Here's how the part is built. I have some questions about the finished solid (model axes, mm). A direction names the side the tool comes from. Give positions to 0.01 mm unless a question says otherwise; leave off trailing zeros. Order: outer loops, then holes, each group sorted by start corner. A loop starts at its lowest first (then second) coordinate and runs counter-clockwise, first axis right, second up.
from build123d import *

# Parameters (mm, degrees)
F0_W         = 40.64
F0_H         = 5.08
F1_DEPTH     = 6.35
F3_DEPTH     = 7.62
F4_R         = 1.26999
F5_T1_DEPTH  = 6.35
F5_T3_DEPTH  = 85.09
F5_T5_DEPTH  = 72.39
F5_T8_ANGLE  = 90
F5_T10_ANGLE = 90
F5_T12_ANGLE = 90
F5_T14_ANGLE = 90
F6_R         = 5.07999
F7_R         = 2.54


# Not quite as in the source:
# - a fillet or chamfer that OpenCascade refuses, or shapes differently, is made with other operations: its cross-section is extruded or revolved along the edge and cut away or added
# - a fillet or chamfer is up to 0.001 mm smaller than in the source, because OpenCascade refuses the exact size


with BuildPart() as f1:
    # F0 (on Front) → F1 (new body)
    with BuildSketch(Plane.XZ):
        with BuildLine():
            ThreePointArc((-31.75, 19.05), (-45.2203841816, 13.4703841816), (-50.8, 0))
            Line((-50.8, 0), (-50.8, -6.35))
            ThreePointArc((-50.8, -6.35), (-48.9401280605, -10.8401280605), (-44.45, -12.7))
            Line((-44.45, -12.7), (27.94, -12.7))
            Line((27.94, -12.7), (27.94, 19.05))
            Line((27.94, 19.05), (20.32, 19.05))
            Line((20.32, 19.05), (-31.75, 19.05))
        make_face()
        Rectangle(F0_W, F0_H, mode=Mode.SUBTRACT)
    extrude(amount=F1_DEPTH)

    # F2 (on face) → F3 (join)
    with BuildSketch(Plane.YZ.offset(27.94)):
        Polygon((-4.445, -5.715), (-3.175, -5.715), (-1.905, -5.715), (-1.905, 12.065), (-4.445, 12.065), align=None)
    extrude(amount=F3_DEPTH)

    # F4 (radius 1.27 in the source; OpenCascade refuses exactly that, so slightly less here)
    f4_edges = [f1.edges().sort_by_distance(p)[0] for p in [
        (35.56, -4.445, 3.175),
        (35.56, -3.175, 12.065),
        (35.56, -1.905, 3.175),
        (35.56, -3.175, -5.715),
    ]]
    fillet(f4_edges, radius=F4_R)

    # F5: fillet of radius 5.08 on 2 edges, made by hand

    # F5_s2 → F5_t1 (cut)
    with BuildSketch(Plane.XY.offset(-6.35)):
        with BuildLine():
            ThreePointArc((-45.72, 0), (-49.3121024484, -1.4878975516), (-50.8, -5.08))
            Line((-50.8, -5.08), (-50.8, 0))
            Line((-50.8, 0), (-45.72, 0))
        make_face()
        with BuildLine():
            ThreePointArc((-45.72, -6.35), (-49.3121024484, -4.8621024484), (-50.8, -1.27))
            Line((-50.8, -1.27), (-50.8, -6.35))
            Line((-50.8, -6.35), (-45.72, -6.35))
        make_face()
    extrude(amount=F5_T1_DEPTH, mode=Mode.SUBTRACT)

    # F5_s4 → F5_t3 (cut)
    with BuildSketch(Plane.YZ.offset(-44.45)):
        with BuildLine():
            ThreePointArc((-5.08, -12.7), (-1.4878975516, -11.2121024484), (0, -7.62))
            Line((0, -7.62), (0, -12.7))
            Line((0, -12.7), (-5.08, -12.7))
        make_face()
        with BuildLine():
            ThreePointArc((-1.27, -12.7), (-4.8621024484, -11.2121024484), (-6.35, -7.62))
            Line((-6.35, -7.62), (-6.35, -12.7))
            Line((-6.35, -12.7), (-1.27, -12.7))
        make_face()
    extrude(amount=F5_T3_DEPTH, mode=Mode.SUBTRACT)

    # F5_s6 → F5_t5 (cut)
    with BuildSketch(Plane.YZ.offset(-31.75)):
        with BuildLine():
            ThreePointArc((0, 13.97), (-1.4878975516, 17.5621024484), (-5.08, 19.05))
            Line((-5.08, 19.05), (0, 19.05))
            Line((0, 19.05), (0, 13.97))
        make_face()
        with BuildLine():
            ThreePointArc((-6.35, 13.97), (-4.8621024484, 17.5621024484), (-1.27, 19.05))
            Line((-1.27, 19.05), (-6.35, 19.05))
            Line((-6.35, 19.05), (-6.35, 13.97))
        make_face()
    extrude(amount=F5_T5_DEPTH, mode=Mode.SUBTRACT)

    # F5_s7 → F5_t8 (revolve, cut)
    with BuildSketch(Plane.XY.offset(-6.35)):
        with BuildLine():
            ThreePointArc((-45.72, -6.35), (-49.3121024484, -4.8621024484), (-50.8, -1.27))
            Line((-50.8, -1.27), (-50.8, -6.35))
            Line((-50.8, -6.35), (-45.72, -6.35))
        make_face()
    revolve(axis=Axis((-44.45, -6.35, -6.35), (0, -1, 0)), revolution_arc=F5_T8_ANGLE, mode=Mode.SUBTRACT)

    # F5_s9 → F5_t10 (revolve, cut)
    with BuildSketch(Plane.YZ.offset(-31.75)):
        with BuildLine():
            ThreePointArc((0, 13.97), (-1.4878975516, 17.5621024484), (-5.08, 19.05))
            Line((-5.08, 19.05), (0, 19.05))
            Line((0, 19.05), (0, 13.97))
        make_face()
    revolve(axis=Axis((-31.75, 0, 0), (0, -1, 0)), revolution_arc=F5_T10_ANGLE, mode=Mode.SUBTRACT)

    # F5_s11 → F5_t12 (revolve, cut)
    with BuildSketch(Plane.XY.offset(-6.35)):
        with BuildLine():
            ThreePointArc((-45.72, 0), (-49.3121024484, -1.4878975516), (-50.8, -5.08))
            Line((-50.8, -5.08), (-50.8, 0))
            Line((-50.8, 0), (-45.72, 0))
        make_face()
    revolve(axis=Axis((-44.45, 0, -6.35), (0, -1, 0)), revolution_arc=F5_T12_ANGLE, mode=Mode.SUBTRACT)

    # F5_s13 → F5_t14 (revolve, cut)
    with BuildSketch(Plane.YZ.offset(-31.75)):
        with BuildLine():
            ThreePointArc((-6.35, 13.97), (-4.8621024484, 17.5621024484), (-1.27, 19.05))
            Line((-1.27, 19.05), (-6.35, 19.05))
            Line((-6.35, 19.05), (-6.35, 13.97))
        make_face()
    revolve(axis=Axis((-31.75, -6.35, 0), (0, -1, 0)), revolution_arc=F5_T14_ANGLE, mode=Mode.SUBTRACT)

    # F6 (radius 5.08 in the source; OpenCascade refuses exactly that, so slightly less here)
    f6_edges = [f1.edges().sort_by_distance(p)[0] for p in [
        (20.32, -3.175, -2.54),
    ]]
    fillet(f6_edges, radius=F6_R)

    # F7
    f7_edges = [f1.edges().sort_by_distance(p)[0] for p in [
        (-20.32, -3.175, -2.54),
    ]]
    fillet(f7_edges, radius=F7_R)


solid = f1.part
Q1. I need wall thicknesses on L1, parallel to X at y = -3.25, z = -1; L2, parallel to Z at x = 31, y = -2 (3 decimals); L3, parallel to Z at x = 19.5, y = -2.25. Which ranges of each line are inside material? Lowest first, please.
Filled sheet:
L1: x = -50.4 to -20.11, 18.88 to 35.56
L2: z = -5.715 to 12.065
L3: z = -11.84 to -0.23, 2.54 to 18.19
Q2. For faces 1 (the face through (31, -3, 12.065)), 2 (the face through (0, -3, 2.54)), 3 (the face through (31, -4.445, 3)), 4 (the face through (31, -1.905, 3)), which set-ups out of +Z, -Z, +X, -X, +Y, -Y let a thin tool reach every point of the face, with its end or its side?
Filled sheet:
face 1: +Z, +X, +Y, -Y
face 2: +Y, -Y
face 3: +Z, -Z, +X, -Y
face 4: +Z, -Z, +X, +Y
Q3. I'm going to push flat-ended pins straight in: P1, Ø1.9, axis at x = -4, y = -4.5, coming from the -Z side; P2, Ø2, axis at x = 31, y = -3.5, coming from the -Z side (3 decimals); P3, Ø1.3, axis at x = 31.5, y = -3, coming from the +Z side (3 decimals). Where does each tip first touch, or does it pass through?
Filled sheet:
P1: stops at z = -12.16
P2: stops at z = -5.715
P3: stops at z = 12.065
Q4. If we section it at A-A on x = -4: List the corners of the cut face in (y, z) for me (3 decimals).
Filled sheet:
outline: (-6.35, -7.62) arc R5.08 ccw to (-3.175, -12.329) arc R5.08 ccw to (0, -7.62) - (0, -2.54) - (-6.35, -2.54) - close; (-6.35, 2.54) - (0, 2.54) - (0, 13.97) arc R5.08 ccw to (-3.175, 18.679) arc R5.08 ccw to (-6.35, 13.97) - close
Q5. Thinking about a two-plate mould opening in X: for faces 5 (the face through (-20.32, -3, 1)), 6 (the face through (31, -3, -5.715)), 7 (the face through (-48.52, -0.84, -3.22)), which applies, released by +X, released by -X, zero draft, split by the parting line, or undercut?
Filled sheet:
face 5: undercut
face 6: zero draft
face 7: released by -X
